Geometry check sheet. Reference: the model listing, model coordinates, mm. Coordinates: 2 decimals unless noted, no trailing zeros. Write each loop counter-clockwise with the first axis right and the second up, starting at its lowest first coordinate (ties: lowest second). Pieces come first, ordered by that corner, then holes. Notation, with made-up numbers: (-27, -29) -> (0, -29) arc R11 ccw to (0, -12) -> close; hole circle Ø6 at (-33.5, 17.25). An arc over 180 degrees is marked (long way). Use a Markdown table: item, result.
```python
from build123d import *

# Parameters (mm, degrees)
F0_R     = 31.75
F0_R_2   = 24.7772994978
F0_R_3   = 19.1989713068
F0_R_4   = 12.7
F1_DEPTH = 44.45
F2_D     = 9.0424


# Not quite as in the source:
# - a fillet or chamfer that OpenCascade refuses, or shapes differently, is made with other operations: its cross-section is extruded or revolved along the edge and cut away or added


with BuildPart() as f1:
    # F0 (on Front) → F1 (new body)
    with BuildSketch(Plane.XZ):
        Circle(F0_R)
        Circle(F0_R_2, mode=Mode.SUBTRACT)
        Circle(F0_R_2)
        Circle(F0_R_3, mode=Mode.SUBTRACT)
        Circle(F0_R_3)
        Circle(F0_R_4, mode=Mode.SUBTRACT)
    extrude(amount=F1_DEPTH)

    # F2 (through all)
    with Locations(Plane(origin=(0, 0, 0), x_dir=(1, 0, 0), z_dir=(0, 1, 0))):
        with Locations((24.7772994978, 0), (0, 24.7772994978), (-24.7772994978, 0), (0, -24.7772994978)):
            Hole(F2_D / 2)

    # F3: chamfer of 5.08 on 4 edges, made by hand

    # F3_s1 → F3_t2 (revolve, cut)
    with BuildSketch(Plane.XY):
        Polygon((12.7, -39.37), (17.78, -44.45), (12.7, -44.45), align=None)
    revolve(axis=Axis((0, -44.45, 0), (0, -1, 0)), mode=Mode.SUBTRACT)

    # F3_s3 → F3_t4 (revolve, cut)
    with BuildSketch(Plane.XY):
        Polygon((26.67, -44.45), (31.75, -39.37), (31.75, -44.45), align=None)
    revolve(axis=Axis((0, -44.45, 0), (0, -1, 0)), mode=Mode.SUBTRACT)

    # F3_s5 → F3_t6 (revolve, cut)
    with BuildSketch(Plane.XY):
        Polygon((12.7, -5.08), (17.78, 0), (12.7, 0), align=None)
    revolve(axis=Axis((0, 0, 0), (0, -1, 0)), mode=Mode.SUBTRACT)

    # F3_s7 → F3_t8 (revolve, cut)
    with BuildSketch(Plane.XY):
        Polygon((26.67, 0), (31.75, -5.08), (31.75, 0), align=None)
    revolve(axis=Axis((0, 0, 0), (0, -1, 0)), mode=Mode.SUBTRACT)


solid = f1.part
```
Item 1: Thickness scan on L1, parallel to Z at x = 0, y = -28; L2, parallel to X at y = -24.5, z = 4; L3, parallel to X at y = -42, z = 10.5. Record the ranges inside material, lowest first. Write a range as [from, to].
Answer block:
| item | result |
|---|---|
| L1 | z = [-31.75, -29.3], [-20.26, -12.7], [12.7, 20.26], [29.3, 31.75] |
| L2 | x = [-31.5, -26.88], [-22.67, -12.05], [12.05, 22.67], [26.88, 31.5] |
| L3 | x = [-27.16, -11.17], [11.17, 27.16] |
Item 2: Section check B-B on x = 0. Record the boundary of the cut face in (y, z), then the cut area to 3 significant figures.
Answer block:
| item | result |
|---|---|
| outline | (-44.45, -20.26) -> (0, -20.26) -> (0, -17.78) -> (-5.08, -12.7) -> (-39.37, -12.7) -> (-44.45, -17.78) -> close; (-44.45, 17.78) -> (-39.37, 12.7) -> (-5.08, 12.7) -> (0, 17.78) -> (0, 20.26) -> (-44.45, 20.26) -> close; (-41.82, -29.3) -> (-39.37, -31.75) -> (-5.08, -31.75) -> (-2.63, -29.3) -> close; (-41.82, 29.3) -> (-2.63, 29.3) -> (-5.08, 31.75) -> (-39.37, 31.75) -> close |
| area | 800 mm^2 |
Item 3: Mould release check, pull along Z, two halves, no side actions. Record for faces 1 (the cylindrical face through (-6.883, -21.985, -30.995)), 2 (the conical face through (-2.82, -4.76, -12.71)), 3 (the cylindrical face through (-20.26, -22.54, -0.2)), 4 (the flat face through (-18, 0, 0)): +Z half, -Z half, draft (parallel to the pull), parting line (faces both ways), or undercut.
Answer block:
| item | result |
|---|---|
| face 1 | parting line |
| face 2 | undercut |
| face 3 | undercut |
| face 4 | draft |
Item 4: Depth check by flat-ended pin: P1, Ø1, axis at y = -17.5, z = 16, coming from the +X side; P2, Ø8, axis at x = -24.78, z = 0, coming from the +Y side (1 decimal); P3, Ø3, axis at x = 12, z = -5.5, coming from the -Y side; P4, Ø2, axis at y = -11.5, z = 16, coming from the -X side. Enter the tip coordinate at first touch or a pass-through.
Answer block:
| item | result |
|---|---|
| P1 | stops at x = 27.71 |
| P2 | passes through |
| P3 | stops at y = -41.37 |
| P4 | stops at x = -27.98 |
Item 5: Section check A-A on z = 0. Record the boundary of the cut face in (x, y), then the cut area to 3 significant figures.
Answer block:
| item | result |
|---|---|
| outline | (-31.75, -39.37) -> (-29.3, -41.82) -> (-29.3, -2.63) -> (-31.75, -5.08) -> close; (-20.26, -44.45) -> (-17.78, -44.45) -> (-12.7, -39.37) -> (-12.7, -5.08) -> (-17.78, 0) -> (-20.26, 0) -> close; (12.7, -39.37) -> (17.78, -44.45) -> (20.26, -44.45) -> (20.26, 0) -> (17.78, 0) -> (12.7, -5.08) -> close; (29.3, -41.82) -> (31.75, -39.37) -> (31.75, -5.08) -> (29.3, -2.63) -> close |
| area | 800 mm^2 |
Item 6: Section check C-C on y = -6.5. Record the boundary of the cut face in (x, z).
Answer block:
| item | result |
|---|---|
| outline | circle Ø63.5 at (0, 0); hole circle Ø9.04 at (-24.78, 0); hole circle Ø25.4 at (0, 0); hole circle Ø9.04 at (0, -24.78); hole circle Ø9.04 at (0, 24.78); hole circle Ø9.04 at (24.78, 0) |
